```python
from build123d import *

# Parameters (mm, degrees)
F0_R      = 12.75
F1_DEPTH  = 2.75
F2_R      = 12
F3_DEPTH  = 4.25
F4_R      = 20
F5_DEPTH  = 6
F6_SIZE2  = 6
F6_SIZE   = 1.5
F7_R      = 12
F8_DEPTH  = 4.25
F9_R      = 20
F10_DEPTH = 6
F11_SIZE2 = 6
F11_SIZE  = 1.5


with BuildPart() as f1:
    # F0 (on Top) → F1 (new body, symmetric)
    with BuildSketch(Plane.XY):
        Circle(F0_R)
    extrude(amount=F1_DEPTH, both=True)

    # F2 (on face) → F3 (join)
    with BuildSketch(Plane.XY.offset(2.75)):
        Circle(F2_R)
    extrude(amount=F3_DEPTH)



with BuildPart() as f5:
    # F4 (on face) → F5 (new body)
    with BuildSketch(Plane(origin=(0, 0, -7), x_dir=(1, 0, 0), z_dir=(0, 0, -1))):
        Circle(F4_R)
    extrude(amount=F5_DEPTH)

    # F6
    f6_edges = [f5.edges().sort_by_distance(p)[0] for p in [
        (-20, 0, -7),
    ]]
    chamfer(f6_edges, length=F6_SIZE, length2=F6_SIZE2)


with BuildPart() as f1_1:
    add(f1.part)

    add(f5.part)  # F8 merges F5
    # F7 (on face) → F8 (join)
    with BuildSketch(Plane(origin=(0, 0, -2.75), x_dir=(1, 0, 0), z_dir=(0, 0, -1))):
        Circle(F7_R)
    extrude(amount=F8_DEPTH)

    # F9 (on face) → F10 (join)
    with BuildSketch(Plane.XY.offset(7)):
        Circle(F9_R)
    extrude(amount=F10_DEPTH)

    # F11
    f11_edges = [f1_1.edges().sort_by_distance(p)[0] for p in [
        (-20, 0, 7),
    ]]
    chamfer(f11_edges, length=F11_SIZE, length2=F11_SIZE2)


solid = f1_1.part
```
Design review of the part built by this model. Coordinates are the model's own, in mm. A direction names the side the tool comes from. Round coordinates to 2 decimals unless told otherwise and drop trailing zeros. Write each loop counter-clockwise with the first axis right and the second up, starting at its lowest first coordinate (ties: lowest second). Pieces come first, ordered by that corner, then holes. Notation, with made-up numbers: (56, 20) -> (112, 20) arc R11 cw to (112, 30) -> close; hole circle Ø10 at (-9, 13). An arc over 180 degrees is marked (long way). Write item = value, one per line. Start each with the question number.
1) Mouldability with a two-part tool opening along Z and no side actions: class faces 3 (the face through (-2.764, -12.447, 0.038)), 4 (the face through (0, 0, 13)), 5 (the face through (-11.341, -8.696, 7.073)), 6 (the face through (0, 0, -13)) as +Z half, -Z half, draft (parallel to the pull), parting line (faces both ways), or undercut.
2) Clearance check with flat-ended pins moving along their axes: pin 1 (6 mm diameter, centred on x = -13.5, z = -0.5, fed in from -Y); pin 2 (6 mm diameter, centred on y = 10.5, z = 4, fed in from +X); pin 3 (6 mm diameter, centred on y = 13.5, z = 4, fed in from -X). State where each tip first meets the part, or that it passes through.
3) Tool access review of faces 1 (the face through (-11.99, -0.53, -4.85)), 2 (the face through (-4.336, 19.524, -10.718)): name each direction out of +Z, -Z, +X, -X, +Y, -Y from which nothing blocks a thin tool from reaching the whole face with its end or side.
4) Take a section at D-D, the plane z = -10. State the section outline as (x, y) points, plus the area to 3 significant figures.
5) Take a section at C-C, the plane z = -5. State the section outline as (x, y) points, plus the area to 3 significant figures.
6) Take a section at A-A, the plane y = 0. State the section outline as (x, z) points.
7) Wall thickness on probe 1 along Z at (x, y) = (6, -11.5); probe 2 along Z at (x, y) = (-0.5, -16); probe 3 along X at (y, z) = (7, -1): over which ranges is each line inside the solid? List them lowest first. Write a range as from..to.
Results list:
q1.face_3 = undercut
q1.face_4 = +Z half
q1.face_5 = undercut
q1.face_6 = -Z half
q2.pin_1 = -7.23
q2.pin_2 = 10.11
q2.pin_3 = -6.82
q3.face_1 = none
q3.face_2 = +Z, -Z
q4.outline = circle Ø40 at (0, 0)
q4.area = 1,260 mm²
q5.outline = circle Ø24 at (0, 0)
q5.area = 452 mm²
q6.outline = (-20, -13) -> (20, -13) -> (20, -8.5) -> (14, -7) -> (12, -7) -> (12, -2.75) -> (12.75, -2.75) -> (12.75, 2.75) -> (12, 2.75) -> (12, 7) -> (14, 7) -> (20, 8.5) -> (20, 13) -> (-20, 13) -> (-20, 8.5) -> (-14, 7) -> (-12, 7) -> (-12, 2.75) -> (-12.75, 2.75) -> (-12.75, -2.75) -> (-12, -2.75) -> (-12, -7) -> (-14, -7) -> (-20, -8.5) -> close
q7.probe_1 = -13..-7, 7..13
q7.probe_2 = -13..-7.5, 7.5..13
q7.probe_3 = -10.66..10.66
